Check sheet for the drawn part. Datum: minimum x, y, z corner. Units: mm. A direction names the side the tool comes from. Round coordinates to 2 decimals unless told otherwise and drop trailing zeros. Loops run counter-clockwise (first coordinate to the right, second up) from the corner with the lowest first, then second, coordinate; pieces in that order, holes last.
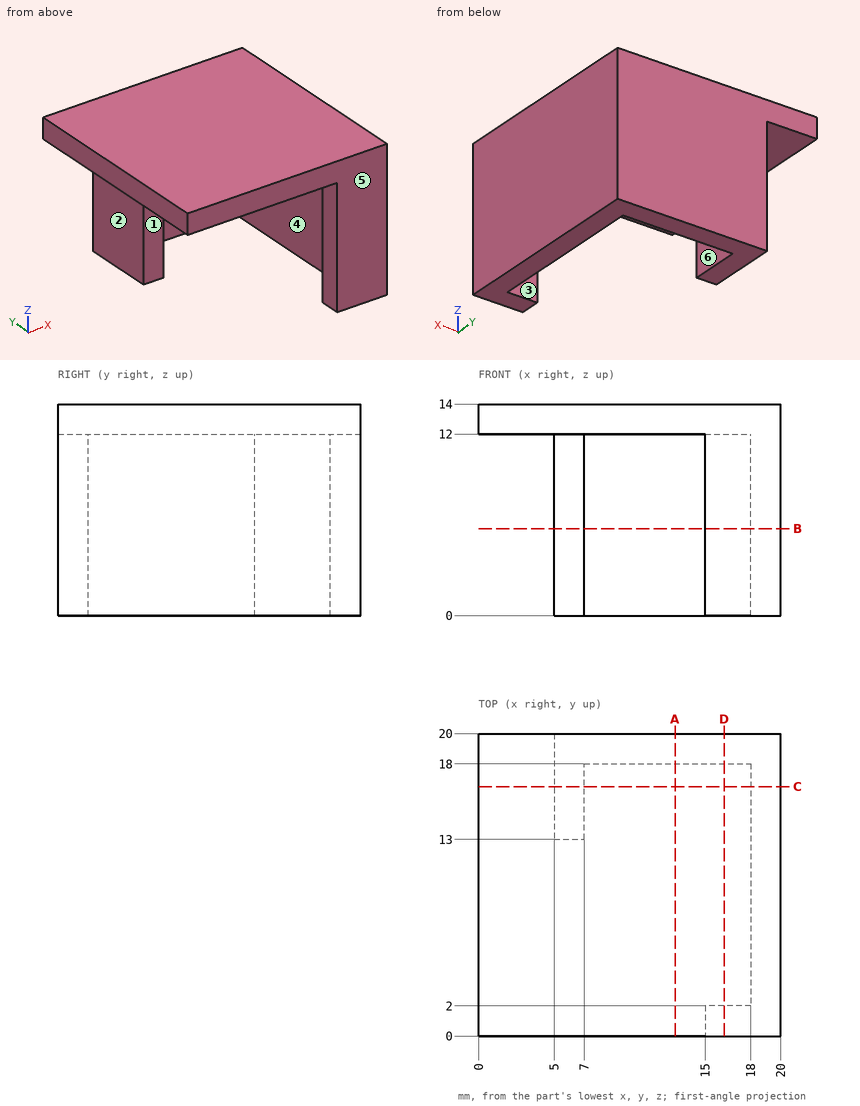
1) Sectioned sample at B-B, the plane z = 5.75. Record the cut outline in (x, y).
Report:
outline: (5, 13) - (7, 13) - (7, 18) - (18, 18) - (18, 2) - (15, 2) - (15, 0) - (20, 0) - (20, 20) - (5, 20) - close
2) Mould release check, pull along Y, two halves, no side actions. Record for the marked faces 1, 2 and 3: +Y half, -Y half, draft (parallel to the pull), parting line (faces both ways), or undercut.
Report:
face 1: -Y half
face 2: draft
face 3: undercut
3) Gauge pin test, flat ends, axial feed: pin 1 (5 mm diameter, centred on x = 14, z = 11.5, fed in from -Y); pin 2 (1.6 mm diameter, centred on y = 1, z = 5.5, fed in from -X); pin 3 (6 mm diameter, centred on y = 13.5, z = 6, fed in from -X); pin 4 (2 mm diameter, centred on x = 6.5, z = 3.5, fed in from -Y). Record the tip position at first contact, or that the pin passes through.
Report:
pin 1: stops at y = 0
pin 2: stops at x = 15
pin 3: stops at x = 5
pin 4: stops at y = 13
4) Access from +Z, -Z, +X, -X, +Y, -Y to the whole of each face (thin tool, end or side, straight path). Record for the marked faces 4, 5 and 6.
Report:
face 4: -Z
face 5: +Z, -Z, +X, -X, -Y
face 6: -Z, -Y
5) Scan lines: line 1 along X through (y, z) = (15.5, 2); line 2 along Z through (x, y) = (13.25, 13); line 3 along X through (y, z) = (3.75, 3.25). Record each from-to range of solid material in increasing order.
Report:
line 1: x = 5 to 7, 18 to 20
line 2: z = 12 to 14
line 3: x = 18 to 20
6) Sectioned sample at D-D, the plane x = 16.25. Record the cut outline in (y, z), then the cut area to 3 significant figures.
Report:
outline: (0, 0) - (2, 0) - (2, 12) - (18, 12) - (18, 0) - (20, 0) - (20, 14) - (0, 14) - close
area: 88.0 mm2
7) Sectioned sample at C-C, the plane y = 16.5. Record the cut outline in (x, z), then the cut area to 3 significant figures.
Report:
outline: (0, 12) - (5, 12) - (5, 0) - (7, 0) - (7, 12) - (18, 12) - (18, 0) - (20, 0) - (20, 14) - (0, 14) - close
area: 88.0 mm2
8) Sectioned sample at A-A, the plane x = 13. Record the cut outline in (y, z).
Report:
outline: (0, 12) - (18, 12) - (18, 0) - (20, 0) - (20, 14) - (0, 14) - close
